Part model, mm, in its own coordinate system. Face numbers are marked on the shaded views. A direction names the side the tool comes from. Round coordinates to 2 decimals unless told otherwise and drop trailing zeros. Loops run counter-clockwise (first coordinate to the right, second up) from the corner with the lowest first, then second, coordinate; pieces in that order, holes last.
(1) Cut at D-D on y = 22.5. List the corners of the cut face in (x, z).
(2) Flat gauge pins, fed straight in: pin 1 (2 mm diameter, centred on x = 123, y = -1, fed in from +Z); pin 2 (6 mm diameter, centred on x = 120, y = -8.5, fed in from -Z); pin 3 (4.5 mm diameter, centred on y = 0, z = -0.5, fed in from +X). Where does each tip first touch, or does it go through?
(3) Tool access for the marked faces 1, 2 and 3: list every direction of +Z, -Z, +X, -X, +Y, -Y with a clear straight run to the whole face (end or side of a thin tool).
(4) Probe probe 1 along Z at (x, y) = (128.5, 0); probe 2 along Z at (x, y) = (77.45, 11.25); probe 3 along X at (y, z) = (23.5, -3). List the from-to ranges inside material, lowest first.
(5) Cut at A-A on y = 11.25. List the corners of the cut face in (x, z), then the cut area to 3 significant figures.
(6) Cut at C-C on x = 124. List the corners of the cut face in (y, z).
(7) Cut at B-B on z = 0. Count the separate pieces of the cut face and the enclosed holes in it, then the cut area to 3 significant figures.
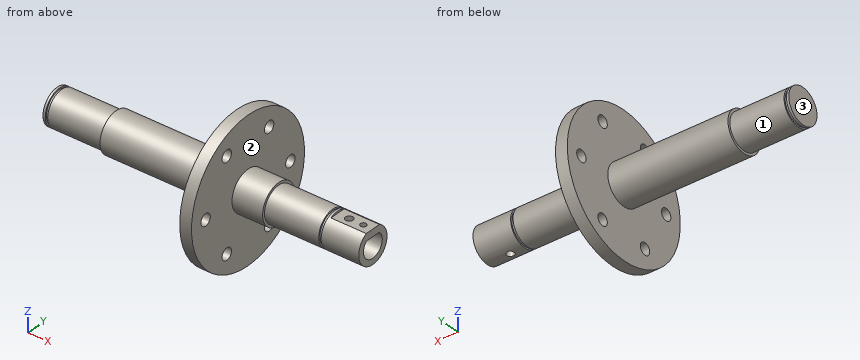
from build123d import *

# Parameters (mm, degrees)
SKETCH_2_R             = 2.5
CUT_EXTRUDE_1_DEPTH    = 88.040220588
CUT_EXTRUDE_2_DEPTH    = 14
CUT_EXTRUDE_START      = -15
CUT_EXTRUDE_3_DEPTH    = 15
SKETCH_5_R             = 1.6
CUT_EXTRUDE_4_DEPTH    = 143.119650207
HOLE_WIZARD_M3_1_D     = 2.5
HOLE_WIZARD_M3_1_DEPTH = 4
HOLE_WIZARD_M3_1_TIP   = 0.751075774
CUT_EXTRUDE_START_2    = 1.03
SKETCH_8_R             = 7.5
SKETCH_8_R_2           = 6.9
CUT_EXTRUDE_5_DEPTH    = 1.03
SKETCH_9_R             = 7.5
SKETCH_9_R_2           = 6.9
CUT_EXTRUDE_6_DEPTH    = 1.03


with BuildPart() as part:
    # 草图1 → 旋转1 (revolve)
    with BuildSketch(Plane.XY, mode=Mode.PRIVATE) as revolve_1_sk:
        Polygon((0, 0), (134, 0), (134, 7.5), (94, 7.5), (94, 8.5), (81, 8.5), (81, 30), (76, 30), (76, 8.5), (25, 8.5), (25, 7.5), (0, 7.5), align=None)
    revolve(revolve_1_sk.sketch.rotate(Axis((0, 0, 0), (1, 0, 0)), 90), axis=Axis((0, 0, 0), (1, 0, 0)))

    # 草图2 → 切除-拉伸1 (cut, through all)
    with BuildSketch(Plane.ZY.offset(-76)):
        with Locations(Location((0, 22.5, 0), (0, 0, 270))):
            Circle(SKETCH_2_R)
        with Locations(Location((19.485571585, 11.25, 0), (0, 0, 270))):
            Circle(SKETCH_2_R)
        with Locations(Location((19.485571585, -11.25, 0), (0, 0, 270))):
            Circle(SKETCH_2_R)
        with Locations(Location((0, -22.5, 0), (0, 0, 270))):
            Circle(SKETCH_2_R)
        with Locations(Location((-19.485571585, -11.25, 0), (0, 0, 270))):
            Circle(SKETCH_2_R)
        with Locations(Location((-19.485571585, 11.25, 0), (0, 0, 270))):
            Circle(SKETCH_2_R)
    extrude(amount=-CUT_EXTRUDE_1_DEPTH, mode=Mode.SUBTRACT)

    # 草图3 → 切除-拉伸2 (cut)
    with BuildSketch(Plane(origin=(134, 0, 0), x_dir=(0, 0, -1), z_dir=(1, 0, 0))):
        with BuildLine():
            Line((-3.570714214, 3.5), (-3.570714214, -3.5))
            ThreePointArc((-3.570714214, -3.5), (5, 0), (-3.570714214, 3.5))
        make_face()
    extrude(amount=-CUT_EXTRUDE_2_DEPTH, mode=Mode.SUBTRACT)

    # 草图4 → 切除-拉伸3 (cut)
    with BuildSketch(Plane(origin=(134, 0, 0), x_dir=(0, 0, -1), z_dir=(1, 0, 0)).offset(CUT_EXTRUDE_START)):
        with BuildLine():
            Line((-6.633249581, 3.5), (-6.633249581, -3.5))
            ThreePointArc((-6.633249581, -3.5), (-7.5, 0), (-6.633249581, 3.5))
        make_face()
    extrude(amount=CUT_EXTRUDE_3_DEPTH, mode=Mode.SUBTRACT)

    # 草图5 → 切除-拉伸4 (cut, through all)
    with BuildSketch(Plane.XY.offset(6.633249581)):
        with Locations((124, 0)):
            Circle(SKETCH_5_R)
    extrude(amount=-CUT_EXTRUDE_4_DEPTH, mode=Mode.SUBTRACT)

    # M3 螺纹孔1
    with Locations(Plane(origin=(130, 0, 6.633249581), x_dir=(1, 0, 0), z_dir=(0, 0, 1))):
        with Locations((0, 0)):
            Hole(HOLE_WIZARD_M3_1_D / 2, depth=HOLE_WIZARD_M3_1_DEPTH)
            with Locations((0, 0, -(HOLE_WIZARD_M3_1_DEPTH + HOLE_WIZARD_M3_1_TIP / 2))):  # 118° drill point
                Cone(0, HOLE_WIZARD_M3_1_D / 2, HOLE_WIZARD_M3_1_TIP, mode=Mode.SUBTRACT)

    # 草图8 → 切除-拉伸5 (cut)
    with BuildSketch(Plane.ZY.offset(-2).offset(CUT_EXTRUDE_START_2)):
        Circle(SKETCH_8_R)
        with Locations(Location((0, 0, 0), (0, 0, 270))):
            Circle(SKETCH_8_R_2, mode=Mode.SUBTRACT)
    extrude(amount=-CUT_EXTRUDE_5_DEPTH, mode=Mode.SUBTRACT)

    # 草图9 → 切除-拉伸6 (cut)
    with BuildSketch(Plane(origin=(117, 0, 0), x_dir=(0, 0, -1), z_dir=(1, 0, 0))):
        with Locations(Location((0, 0, 0), (0, 0, 180))):
            Circle(SKETCH_9_R)
        with Locations(Location((0, 0, 0), (0, 0, 270))):
            Circle(SKETCH_9_R_2, mode=Mode.SUBTRACT)
    extrude(amount=CUT_EXTRUDE_6_DEPTH, mode=Mode.SUBTRACT)


solid = part.part
Final values:
1. outline: (76, -19.84) - (81, -19.84) - (81, -2.5) - (76, -2.5) - close; (76, 2.5) - (81, 2.5) - (81, 19.84) - (76, 19.84) - close
2. pin 1: stops at z = 6.63
2. pin 2: stops at z = -5.1
2. pin 3: stops at x = 120
3. face 1: -X
3. face 2: +X
3. face 3: +Z, -Z, -X, +Y, -Y
4. probe 1: z = -7.5 to -5, 3.57 to 6.63
4. probe 2: z = -27.81 to -21.99, -16.99 to 16.99, 21.99 to 27.81
4. probe 3: x = 76 to 81
5. outline: (76, -27.81) - (81, -27.81) - (81, -21.99) - (76, -21.99) - close; (76, -16.99) - (81, -16.99) - (81, 16.99) - (76, 16.99) - close; (76, 21.99) - (81, 21.99) - (81, 27.81) - (76, 27.81) - close
5. area: 228 mm2
6. outline: (-3.5, 3.57) - (-1.6, 3.57) - (-1.6, 6.63) - (-3.5, 6.63) arc R7.5 ccw to (-1.6, -7.33) - (-1.6, -4.74) arc R5 cw to start; (1.6, -7.33) arc R7.5 ccw to (3.5, 6.63) - (1.6, 6.63) - (1.6, 3.57) - (3.5, 3.57) arc R5 cw to (1.6, -4.74) - close
7. separate pieces: 3
7. enclosed holes: 0
7. area: 2,170 mm2
